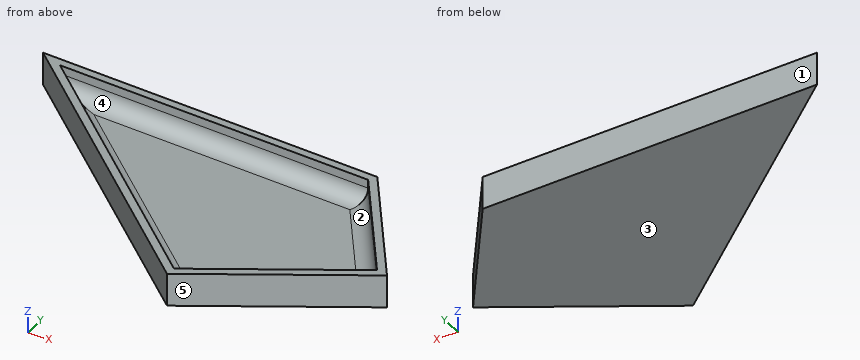
from build123d import *

# Parameters (mm, degrees)
F1_DEPTH = 10.16
F2_T     = -2.5
F3_R     = 5


with BuildPart() as f1:
    # F0 (on Top) → F1 (new body)
    with BuildSketch(Plane.XY):
        Polygon((4.6977261081, 7.2870254517), (-101.8753126264, 11.4898011088), (-18.5698159039, -61.3032579422), (31.5232016146, -31.4628481865), align=None)
    extrude(amount=F1_DEPTH)

    # F2
    f2_openings = [f1.faces().sort_by_distance(p)[0] for p in [
        (-26.57097, -18.043029, 10.16),
    ]]
    offset(amount=F2_T, openings=f2_openings)

    # F3
    f3_edges = [f1.edges().sort_by_distance(p)[0] for p in [
        (-45.772655, 6.775414, 2.5),
        (-56.594272, -24.757201, 2.5),
        (4.826641, -44.456029, 2.5),
        (15.648258, -12.923414, 2.5),
    ]]
    fillet(f3_edges, radius=F3_R)


solid = f1.part
Could you check a few things on this model? Use its own coordinates, in mm. Face numbers are marked on the shaded views. A direction names the side the tool comes from. Round coordinates to 2 decimals unless told otherwise and drop trailing zeros. Order: outer loops, then holes, each group sorted by start corner. A loop starts at its lowest first (then second) coordinate and runs counter-clockwise, first axis right, second up.
(1) Imagine slicing it at A-A (z = 5). Write out the boundary of the cut face in (x, y), plus the area to 3 significant figures.
Response values:
outline: (-101.88, 11.49) - (-18.57, -61.3) - (31.52, -31.46) - (4.7, 7.29) - close; hole (-93.03, 7.97) - (-18.22, -57.4) - (26.99, -30.48) - (2.99, 4.18) - close
area: 971 mm2
(2) If we mould it in two halves opening along X, with no side actions, what happens to the marked faces 3, 4 and 5? For each: released by +X, released by -X, zero draft, split by the parting line, or undercut.
Response values:
face 3: zero draft
face 4: undercut
face 5: released by +X
(3) I'm going to push flat-ended pins straight in: pin 1 (1 mm diameter, centred on x = 7.5, y = -14.5, fed in from -Z); pin 2 (2 mm diameter, centred on x = -7, y = -2.5, fed in from +Z); pin 3 (1.5 mm diameter, centred on x = 18, z = 7.5, fed in from -Y); pin 4 (4 mm diameter, centred on y = -36.5, z = 3, fed in from +X). Where does each tip first touch, or does it pass through?
Response values:
pin 1: stops at z = 0
pin 2: stops at z = 2.5
pin 3: stops at y = -39.97
pin 4: stops at x = 26.42
(4) Please list where these lines run through material, in increasing order: line 1 along X through (y, z) = (-37, 9); line 2 along Z through (x, y) = (4.5, -20); line 3 along Y through (x, z) = (-40, 8).
Response values:
line 1: x = -46.38 to -42.58, 17.34 to 22.23
line 2: z = 0 to 2.5
line 3: y = -42.58 to -39.26, 6.55 to 9.05
(5) Which directions (+Z, -Z, +X, -X, +Y, -Y) give clear straight access to the entire face, cutting with the end or side of a thin tool? Please do the marked faces 1 and 2.
Response values:
face 1: +Z, -Z, +X, +Y
face 2: +Z
